from build123d import *

# Parameters (mm, degrees)
F0_R     = 5
F1_DEPTH = 9
F2_R     = 14.99999


# Not quite as in the source:
# - a fillet or chamfer is up to 0.001 mm smaller than in the source, because OpenCascade refuses the exact size


with BuildPart() as f1:
    # F0 (on Front) → F1 (new body, symmetric)
    with BuildSketch(Plane.XZ):
        Polygon((0, 15), (15, 0), (30, 0), (30, 20), (15, 30), (0, 30), align=None)
        with Locations((15, 15)):
            Circle(F0_R, mode=Mode.SUBTRACT)
    extrude(amount=F1_DEPTH, both=True)

    # F2 (radius 15 in the source; OpenCascade refuses exactly that, so slightly less here)
    f2_edges = [f1.edges().sort_by_distance(p)[0] for p in [
        (0, 0, 30),
    ]]
    fillet(f2_edges, radius=F2_R)


solid = f1.part
The model under review builds one solid part; all positions refer to its coordinate system, in mm. Coordinates: 2 decimals unless noted, no trailing zeros. Order: outer loops, then holes, each group sorted by start corner. A loop starts at its lowest first (then second) coordinate and runs counter-clockwise, first axis right, second up. Notation, with made-up numbers: (7, -17) -> (18, -17) arc R10 ccw to (18, -13) -> close; hole circle Ø3 at (-2, 70). An arc over 180 degrees is marked (long way). Answer in a Markdown table with one row per item.
(1) Insertion check: pin 1 (1.5 mm diameter, centred on y = 3.5, z = 21, fed in from -X); pin 2 (4 mm diameter, centred on x = 4.5, y = 5.5, fed in from -Z); pin 3 (5 mm diameter, centred on y = -4.5, z = 24, fed in from +X). Each pin has a flat end and moves straight along its axis. Give the tip position at first contact, or say it passes through.
Answers:
| item | result |
|---|---|
| pin 1 | x = 0.95 |
| pin 2 | z = 8.5 |
| pin 3 | x = 27.75 |
(2) Consider section C-C (z = 17.5). Write out the cut boundary in (x, y).
Answers:
| item | result |
|---|---|
| outline | (0.21, -9) -> (10.67, -9) -> (10.67, 9) -> (0.21, 9) -> close; (19.33, -9) -> (30, -9) -> (30, 9) -> (19.33, 9) -> close |
(3) Wall thickness on line 1 along Z through (x, y) = (15, 4); line 2 along X through (y, z) = (6, 11.5); line 3 along X through (y, z) = (6.25, 11): over which ranges is each line inside the solid? List them lowest first.
Answers:
| item | result |
|---|---|
| line 1 | 0 to 10, 20 to 30 |
| line 2 | 3.5 to 11.43, 18.57 to 30 |
| line 3 | 4 to 12, 18 to 30 |
(4) The part is to be moulded in two halves that separate along Z. For faces 1 (the flat face through (22.605, -0.126, 24.93)), 2 (the cylindrical face through (17.307, 0.126, 10.564)), 3 (the flat face through (21, -9, 15)), say which applies: +Z half, -Z half, draft (parallel to the pull), parting line (faces both ways), or undercut.
Answers:
| item | result |
|---|---|
| face 1 | +Z half |
| face 2 | undercut |
| face 3 | draft |
(5) Consider section D-D (z = 9). Write out the cut boundary in (x, y).
Answers:
| item | result |
|---|---|
| outline | (6, -9) -> (30, -9) -> (30, 9) -> (6, 9) -> close |
(6) Consider section B-B (x = 19). Write out the cut boundary in (y, z).
Answers:
| item | result |
|---|---|
| outline | (-9, 0) -> (9, 0) -> (9, 12) -> (-9, 12) -> close; (-9, 18) -> (9, 18) -> (9, 27.33) -> (-9, 27.33) -> close |
